```python
from build123d import *

# Parameters (mm, degrees)
SKETCH_R     = 3
SKETCH_R_2   = 5.5
PAD_DEPTH    = 6
PAD001_DEPTH = 6
FILLET_R     = 2
FILLET001_R  = 1
FILLET002_R  = 1
FILLET003_R  = 1


with BuildPart() as part:
    # Sketch → Pad (new body)
    with BuildSketch(Plane.XZ):
        with BuildLine():
            ThreePointArc((-12.548712, 10), (-16.045877, 0), (-12.548712, -10))
            Line((-1.64, -5), (-12.548712, -10))
            Line((81.949241, -23.66356), (-1.64, -5))
            ThreePointArc((81.949241, -23.66356), (93.754695, -20.924986), (99, -10))
            Line((99, -10), (99, 10))
            ThreePointArc((99, 10), (93.025256, 16.570316), (85.918468, 11.244888))
            ThreePointArc((78.36, 5), (83.262272, 6.763181), (85.918468, 11.244888))
            Line((78.36, 5), (-1.64, 5))
            Line((-1.64, 5), (-12.548712, 10))
        make_face()
        with Locations((92.4, 10)):
            Circle(SKETCH_R, mode=Mode.SUBTRACT)
        with Locations((85, -10)):
            Circle(SKETCH_R_2, mode=Mode.SUBTRACT)
    extrude(amount=PAD_DEPTH)

    # Sketch004 (on Face13 of Pad) → Pad001 (join)
    with BuildSketch(Plane.XZ.offset(6)):
        Polygon((81.14045, -22.447344), (90.934021, -21.502348), (90.934021, -30.866373), (92.566284, -32.155006), (92.652191, -33.787262), (86.037239, -33.787262), align=None)
    extrude(amount=-PAD001_DEPTH)

    # Fillet
    fillet_edges = [part.edges().sort_by_distance(p)[0] for p in [
        (86.037239, -3, -33.787262),
    ]]
    fillet(fillet_edges, radius=FILLET_R)

    # Fillet001
    fillet001_edges = [part.edges().sort_by_distance(p)[0] for p in [
        (92.652191, -3, -33.787262),
    ]]
    fillet(fillet001_edges, radius=FILLET001_R)

    # Fillet002
    fillet002_edges = [part.edges().sort_by_distance(p)[0] for p in [
        (92.566284, -3, -32.155006),
    ]]
    fillet(fillet002_edges, radius=FILLET002_R)

    # Fillet003
    fillet003_edges = [part.edges().sort_by_distance(p)[0] for p in [
        (90.934021, -3, -30.866373),
    ]]
    fillet(fillet003_edges, radius=FILLET003_R)


solid = part.part
```
The model under review builds one solid part; all positions refer to its coordinate system, in mm. A direction names the side the tool comes from. Coordinates: 2 decimals unless noted, no trailing zeros. Write each loop counter-clockwise with the first axis right and the second up, starting at its lowest first coordinate (ties: lowest second). Pieces come first, ordered by that corner, then holes.
1) We need section A-A on y = -4.2. State the section outline as (x, z) points.
2) To check wall thickness, follow probe 1 along Z at (x, y) = (92.4, -4.4); probe 2 along Z at (x, y) = (85, -3.7); probe 3 along Z at (x, y) = (75.5, -1.75). State the ranges of each line that lie inside material, in increasing order.
3) We need section D-D on x = 63. State the section outline as (y, z) points.
4) Clearance check with a flat-ended pin moving along its axis: pin 1 Ø1.8 at (y, z) = (-2.5, -27.5) entering from +X. State where the tip first meets the part, or that it passes through.
5) We need section C-C on x = 44. State the section outline as (y, z) points.
6) The part is to be moulded in two halves that separate along Z. For faces 1 (the face through (83.205, -2.958, 6.716)), 2 (the face through (90, -3, 8.2)), 3 (the face through (40.581, -2.958, -14.427)), 4 (the face through (-16.045, -2.958, 0.151)), say which applies: pulls with the +Z half, pulls with the -Z half, needs draft (parallel to the pull), parting line crosses it, or undercut.
7) We need section B-B on z = -12. State the section outline as (x, y) points, then the cut area to 3 significant figures.
8) Machinability: for faces 5 (the face through (-7.018, -2.958, 7.465)), 6 (the face through (-7.018, -2.958, -7.465)), 7 (the face through (83.603, -3.042, -28.15)), 8 (the face through (90.934, -3, -26)), which of the approach directions +Z, -Z, +X, -X, +Y, -Y give a long, thin tool a straight path to every point of the face, cutting with its end or side? Answer none if there is none.
Answer list:
1. outline: (-12.55, -10) - (-1.64, -5) - (81.64, -23.59) - (85.52, -32.58) arc R2 ccw to (87.35, -33.79) - (91.6, -33.79) arc R1 ccw to (92.6, -32.73) - (92.59, -32.61) arc R1 ccw to (92.21, -31.87) - (91.31, -31.17) arc R1 cw to (90.93, -30.38) - (90.93, -22.68) arc R14 ccw to (99, -10) - (99, 10) arc R6.6 ccw to (85.92, 11.24) arc R7.7 cw to (78.36, 5) - (-1.64, 5) - (-12.55, 10) arc R16.05 ccw to start; hole circle Ø11 at (85, -10); hole circle Ø6 at (92.4, 10)
2. probe 1: z = -33.38 to -32.07, -21.88 to 7, 13 to 16.6
2. probe 2: z = -31.39 to -15.5, -4.5 to 8.8
2. probe 3: z = -22.22 to 5
3. outline: (-6, -19.43) - (0, -19.43) - (0, 5) - (-6, 5) - close
4. pin 1: stops at x = 90.93
5. outline: (-6, -15.19) - (0, -15.19) - (0, 5) - (-6, 5) - close
6. face 1: pulls with the +Z half
6. face 2: undercut
6. face 3: pulls with the -Z half
6. face 4: parting line crosses it
7. outline: (29.71, -6) - (79.88, -6) - (79.88, 0) - (29.71, 0) - close; (90.12, -6) - (98.86, -6) - (98.86, 0) - (90.12, 0) - close
7. area: 353 mm2
8. face 5: +Z, +Y, -Y
8. face 6: -Z, +Y, -Y
8. face 7: -Z, -X, +Y, -Y
8. face 8: +X, +Y, -Y
